from build123d import *

# Parameters (mm, degrees)
EXTRUDE_1_DEPTH     = 30
SKETCH_2_R          = 1.6
CUT_EXTRUDE_1_DEPTH = 3.2
SKETCH_4_W          = 3.9
SKETCH_4_H          = 19.3
CUT_EXTRUDE_2_DEPTH = 23
SKETCH_5_W          = 3.9
SKETCH_5_H          = 19.3
CUT_EXTRUDE_3_DEPTH = 23
SKETCH_6_W          = 6.9
SKETCH_6_H          = 4.9
CUT_EXTRUDE_4_DEPTH = 20


with BuildPart() as part:
    # 草图1 → 凸台-拉伸1 (new body)
    with BuildSketch(Plane.XY):
        with BuildLine():
            Line((-10.1, 14.1), (10.1, 14.1))
            ThreePointArc((10.1, 14.1), (13.246625176, 12.796625176), (14.55, 9.65))
            Line((14.55, 9.65), (14.55, -9.65))
            ThreePointArc((14.55, -9.65), (13.246625176, -12.796625176), (10.1, -14.1))
            Line((10.1, -14.1), (-10.1, -14.1))
            ThreePointArc((-10.1, -14.1), (-13.246625176, -12.796625176), (-14.55, -9.65))
            Line((-14.55, -9.65), (-14.55, 9.65))
            ThreePointArc((-14.55, 9.65), (-13.246625176, 12.796625176), (-10.1, 14.1))
        make_face()
    extrude(amount=EXTRUDE_1_DEPTH)

    # 草图2 → 切除-拉伸1 (cut)
    with BuildSketch(Plane(origin=(14.55, 0, 0), x_dir=(0, 0, -1), z_dir=(1, 0, 0))):
        with Locations(Location((-27, -5, 0), (0, 0, 90))):
            Circle(SKETCH_2_R)
        with Locations(Location((-22, -5, 0), (0, 0, 90))):
            Circle(SKETCH_2_R)
        with Locations(Location((-17, -5, 0), (0, 0, 90))):
            Circle(SKETCH_2_R)
        with Locations(Location((-22, 5, 0), (0, 0, 90))):
            Circle(SKETCH_2_R)
        with Locations(Location((-17, 5, 0), (0, 0, 90))):
            Circle(SKETCH_2_R)
        with Locations(Location((-27, 5, 0), (0, 0, 90))):
            Circle(SKETCH_2_R)
    cut_extrude_1 = extrude(amount=-CUT_EXTRUDE_1_DEPTH, mode=Mode.SUBTRACT)

    # 镜向1: 切除-拉伸1 across plane
    add(cut_extrude_1.mirror(Plane(origin=(0, 0, 0), x_dir=(0, 0, 1), z_dir=(1, 0, 0))), mode=Mode.SUBTRACT)

    # 草图4 → 切除-拉伸2 (cut)
    with BuildSketch(Plane(origin=(14.55, 0, 0), x_dir=(0, 0, -1), z_dir=(1, 0, 0))):
        with Locations((-4.45, 0.45)):
            Rectangle(SKETCH_4_W, SKETCH_4_H)
    extrude(amount=-CUT_EXTRUDE_2_DEPTH, mode=Mode.SUBTRACT)

    # 草图5 → 切除-拉伸3 (cut)
    with BuildSketch(Plane.ZY.offset(14.55)):
        with Locations((10.35, 0.45)):
            Rectangle(SKETCH_5_W, SKETCH_5_H)
    extrude(amount=-CUT_EXTRUDE_3_DEPTH, mode=Mode.SUBTRACT)

    # 草图6 → 切除-拉伸4 (cut)
    with BuildSketch(Plane(origin=(0, 0, 0), x_dir=(-1, 0, 0), z_dir=(0, 0, -1))):
        with Locations((0, -11.65)):
            Rectangle(SKETCH_6_W, SKETCH_6_H)
    extrude(amount=-CUT_EXTRUDE_4_DEPTH, mode=Mode.SUBTRACT)


solid = part.part
Model file for the job. Use its own axes, mm. A direction names the side the tool comes from. Give positions to 0.01 mm unless a question says otherwise; leave off trailing zeros. Order: outer loops, then holes, each group sorted by start corner. A loop starts at its lowest first (then second) coordinate and runs counter-clockwise, first axis right, second up. Notation, with made-up numbers: (-14.75, -37.5) - (4.25, -37.5) arc R22 cw to (4.25, -2.5) - close; hole circle Ø11 at (54.25, 62). An arc over 180 degrees is marked (long way). Return JSON: item names as keys, results as strings.
1) Cut at A-A, the plane x = 6.75. Give the cut face in (y, z).
Geometry says:
{"outline": "(-14.1, 0) - (14.1, 0) - (14.1, 30) - (-14.1, 30) - close; hole (-9.2, 2.5) - (10.1, 2.5) - (10.1, 6.4) - (-9.2, 6.4) - close; hole (-9.2, 8.4) - (10.1, 8.4) - (10.1, 12.3) - (-9.2, 12.3) - close"}
2) Cut at D-D, the plane x = -2.75. Give the cut face in (y, z).
Geometry says:
{"outline": "(-14.1, 20) - (-9.2, 20) - (-9.2, 12.3) - (10.1, 12.3) - (10.1, 8.4) - (-9.2, 8.4) - (-9.2, 6.4) - (10.1, 6.4) - (10.1, 2.5) - (-9.2, 2.5) - (-9.2, 0) - (14.1, 0) - (14.1, 30) - (-14.1, 30) - close"}
3) Cut at B-B, the plane y = 0. Give the cut face in (x, z).
Geometry says:
{"outline": "(-14.55, 0) - (14.55, 0) - (14.55, 2.5) - (-8.45, 2.5) - (-8.45, 6.4) - (14.55, 6.4) - (14.55, 30) - (-14.55, 30) - (-14.55, 12.3) - (8.45, 12.3) - (8.45, 8.4) - (-14.55, 8.4) - close"}
4) Probe line 1 (Z direction, x = -12.75, y = -5); line 2 (Z direction, x = -1, y = -8.25); line 3 (Z direction, x = 12.55, y = 5). List the from-to ranges inside material, lowest first. Write a range as from..to.
Geometry says:
{"line 1": "0..8.4, 12.3..15.4, 18.6..20.4, 23.6..25.4, 28.6..30", "line 2": "0..2.5, 6.4..8.4, 12.3..30", "line 3": "0..2.5, 6.4..15.4, 18.6..20.4, 23.6..25.4, 28.6..30"}
5) 3-axis set-ups, long thin cutter, end or side, ignore diameter. For faces 1 (the flat face through (0, -9.2, 7)), 2 (the flat face through (-11.35, -5, 22)), 3 (the flat face through (11.35, 5, 27)): which of +Z, -Z, +X, -X, +Y, -Y reach the whole face in a straight line?
Geometry says:
{"face 1": "-Z, -Y", "face 2": "-X", "face 3": "+X"}
6) Cut at C-C, the plane z = 21. Give the cut face in (x, y).
Geometry says:
{"outline": "(-14.55, -9.65) arc R4.45 ccw to (-10.1, -14.1) - (10.1, -14.1) arc R4.45 ccw to (14.55, -9.65) - (14.55, -6.25) - (11.35, -6.25) - (11.35, -3.75) - (14.55, -3.75) - (14.55, 3.75) - (11.35, 3.75) - (11.35, 6.25) - (14.55, 6.25) - (14.55, 9.65) arc R4.45 ccw to (10.1, 14.1) - (-10.1, 14.1) arc R4.45 ccw to (-14.55, 9.65) - (-14.55, 6.25) - (-11.35, 6.25) - (-11.35, 3.75) - (-14.55, 3.75) - (-14.55, -3.75) - (-11.35, -3.75) - (-11.35, -6.25) - (-14.55, -6.25) - close"}
7) Pull direction Z, two halves, no side cores. Call faces 4 (the flat face through (0, 0, 30)), 5 (the cylindrical face through (13.281, -12.762, 14.79)), 6 (the flat face through (-11.35, 5, 22)), 7 (the flat face through (-6, -9.2, 4)): pulls with the +Z half, pulls with the -Z half, needs draft (parallel to the pull), parting line crosses it, or undercut.
Geometry says:
{"face 4": "pulls with the +Z half", "face 5": "needs draft", "face 6": "undercut", "face 7": "undercut"}
8) Flat gauge pins, fed straight in: P1, Ø1, axis at y = 5, z = 27, coming from the -X side; P2, Ø2, axis at x = -1.5, z = 14.5, coming from the -Y side; P3, Ø3, axis at y = -5, z = 27, coming from the +X side. Where does each tip first touch, or does it go through?
Geometry says:
{"P1": "x = -11.35", "P2": "y = -9.2", "P3": "x = 11.35"}
